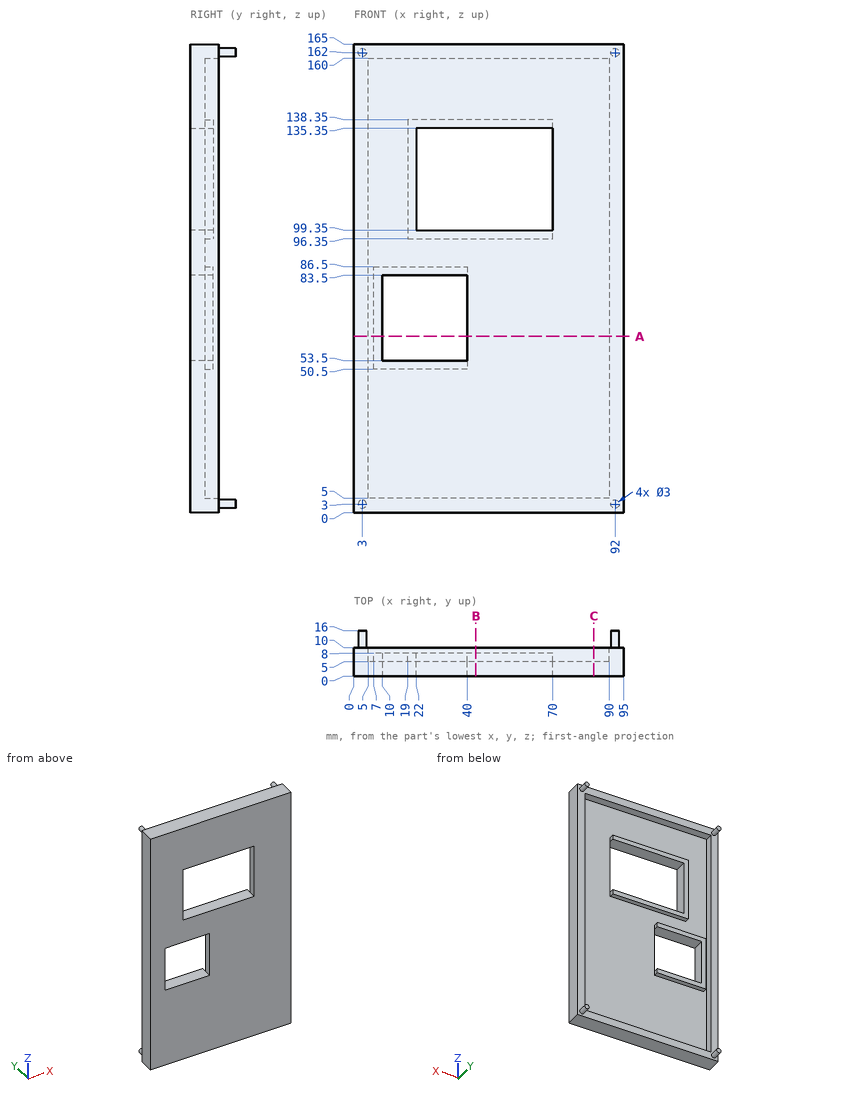
Geometry: see drawing. Coordinates: mm, zero at the bounding-box minimum. Round coordinates to 2 decimals unless told otherwise and drop trailing zeros. Loops run counter-clockwise (first coordinate to the right, second up) from the corner with the lowest first, then second, coordinate; pieces in that order, holes last. Notation, with made-up numbers: M -39,66 L -2,66 A8 ccw -2,70 Z; hole C -38,35.5 d11. An arc over 180 degrees is marked long. Use a Markdown table: item, result. Add a question column.
1. Contact query for a flat-ended pin moving along its axis: P1, Ø16.5, axis at x = 31.5, z = 61, coming from the +Y side. Output: stop coordinate, or through.
2. Line query: line 1 (Z direction, x = 37, y = 7.75); line 2 (Z direction, x = 10.5, y = 5.75); line 3 (Z direction, x = 55, y = 6.5). Output: solid intervals per line, ascending.
3. Section query B-B on x = 43. Return the cut outline in (y, z).
4. Section query A-A on z = 62. Return the cut outline in (x, y), then the cut area to 3 significant figures.
5. Section query C-C on x = 84.5. Return the cut outline in (y, z).
Reported:
| question | item | result |
|---|---|---|
| 1 | P1 | stops at y = 8 |
| 2 | line 1 | z = 0 to 5, 50.5 to 53.5, 83.5 to 86.5, 96.35 to 99.35, 135.35 to 138.35, 160 to 165 |
| 2 | line 2 | z = 0 to 5, 50.5 to 53.5, 83.5 to 86.5, 160 to 165 |
| 2 | line 3 | z = 0 to 5, 96.35 to 99.35, 135.35 to 138.35, 160 to 165 |
| 3 | outline | M 0,0 L 10,0 L 10,5 L 5,5 L 5,96.35 L 8,96.35 L 8,99.35 L 0,99.35 Z; M 0,135.35 L 8,135.35 L 8,138.35 L 5,138.35 L 5,160 L 10,160 L 10,165 L 0,165 Z |
| 4 | outline | M 0,0 L 10,0 L 10,8 L 7,8 L 7,5 L 5,5 L 5,10 L 0,10 Z; M 40,0 L 95,0 L 95,10 L 90,10 L 90,5 L 40,5 Z |
| 4 | area | 384 mm² |
| 5 | outline | M 0,0 L 10,0 L 10,5 L 5,5 L 5,160 L 10,160 L 10,165 L 0,165 Z |
